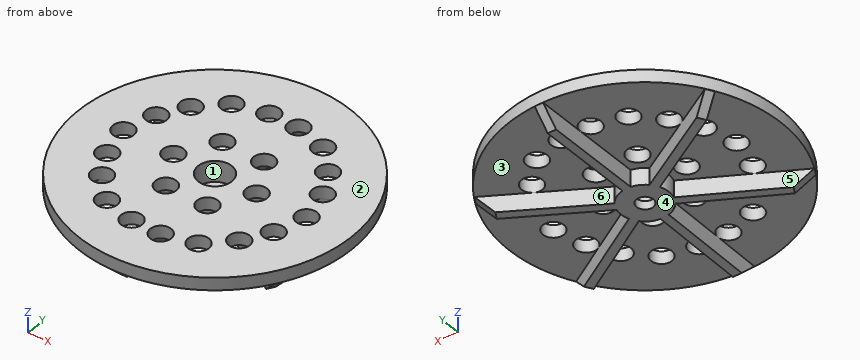
Autodesk Fusion 360 part; units mm, degrees
sketch "Skizze1" plane through (0, 0, 0) normal (0, 0, 1) x (1, 0, 0)
  circle A0 centre (0, 0) radius 32.5
  dimension "d1" = 65
extrude "Extrusion1" add sketch "Skizze1" along normal blind 3
sketch "Skizze2" plane through (0, 0, 0) normal (0, 0, -1) x (1, 0, 0)
  circle A0 centre (0, 0) radius 32.5
  circle A1 centre (0, 0) radius 5.75
  dimension "d4" = 11.5
extrude "Extrusion2" add sketch "Skizze2" along normal blind 4 contours A1
hole "Bohrung1" at (0, 0, 3) direction (0, 0, -1) diameter 4 depth 99 tip angle 118 counterbore diameter 8 counterbore depth 5
sketch "Skizze3" plane through (0, 0, 3) normal (0, 0, 1) x (-1, 0, 0)
  circle A0 centre (0, 0) radius 4
  circle A1 centre (0, 0) radius 32.5
  circle A2 centre (-10, 0.0001) radius 2.5
  circle A3 centre (-22, 0) radius 2.5
  circle A4 centre (-20, 7.5) radius 2.5
  circle A5 centre (-20, -7.5) radius 2.5
  circle A6 centre (-5, -8.6602) radius 2.5
  circle A7 centre (-16.4952, -13.5705) radius 2.5
  circle A8 centre (-11, -19.0526) radius 2.5
  circle A9 centre (-3.5048, -21.0705) radius 2.5
  circle A10 centre (5, -8.6603) radius 2.5
  circle A11 centre (3.5048, -21.0705) radius 2.5
  circle A12 centre (11, -19.0526) radius 2.5
  circle A13 centre (16.4952, -13.5705) radius 2.5
  circle A14 centre (10, -0.0001) radius 2.5
  circle A15 centre (20, -7.5) radius 2.5
  circle A16 centre (22, 0) radius 2.5
  circle A17 centre (20, 7.5) radius 2.5
  circle A18 centre (5, 8.6602) radius 2.5
  circle A19 centre (16.4952, 13.5705) radius 2.5
  circle A20 centre (11, 19.0526) radius 2.5
  circle A21 centre (3.5048, 21.0705) radius 2.5
  circle A22 centre (-5, 8.6603) radius 2.5
  circle A23 centre (-3.5048, 21.0705) radius 2.5
  circle A24 centre (-11, 19.0526) radius 2.5
  circle A25 centre (-16.4952, 13.5705) radius 2.5
  dimension "d12" = 5
  dimension "d13" = 10
  dimension "d14" = 5
  dimension "d15" = 12
  dimension "d18" = 5
  dimension "d19" = 5
  dimension "d21" = 360
extrude "Extrusion3" cut sketch "Skizze3" against normal blind 26 contours A2 | A3 | A4 | A5 | A6 | A7 | A8 | A9 | A10 | A11 | A12 | A13 | A14 | A15 | A16 | A17 | A18 | A19 | A20 | A21 | A22 | A23 | A24 | A25
sketch "Skizze4" plane through (0, 0, 0) normal (0, 0, -1) x (1, 0, 0)
  circle A0 centre (3.5048, -21.0705) radius 2.5
  circle A1 centre (22, 0) radius 2.5
  circle A2 centre (11, 19.0526) radius 2.5
  circle A3 centre (-5, -8.6603) radius 2.5
  circle A4 centre (-22, 0) radius 2.5
  circle A5 centre (-11, 19.0526) radius 2.5
  circle A6 centre (-5, 8.6602) radius 2.5
  circle A7 centre (-10, -0.0001) radius 2.5
  circle A8 centre (5, -8.6602) radius 2.5
  circle A9 centre (16.4952, 13.5705) radius 2.5
  circle A10 centre (20, -7.5) radius 2.5
  circle A11 centre (-3.5048, -21.0705) radius 2.5
  circle A12 centre (11, -19.0526) radius 2.5
  circle A13 centre (20, 7.5) radius 2.5
  circle A14 centre (10, 0.0001) radius 2.5
  circle A15 centre (-11, -19.0526) radius 2.5
  circle A16 centre (-20, 7.5) radius 2.5
  circle A17 centre (-3.5048, 21.0705) radius 2.5
  circle A18 centre (-16.4952, 13.5705) radius 2.5
  circle A19 centre (-16.4952, -13.5705) radius 2.5
  circle A20 centre (-20, -7.5) radius 2.5
  circle A21 centre (3.5048, 21.0705) radius 2.5
  circle A22 centre (16.4952, -13.5705) radius 2.5
  circle A23 centre (5, 8.6603) radius 2.5
  circle A24 centre (0, 0) radius 5.75
  circle A25 centre (0, 0) radius 32.5
  line L0 (1, -32.4807) -> (-1, -32.4807)
  line L1 (-1, -32.4807) -> (-1, -5)
  line L2 (-1, -5) -> (1, -5)
  line L3 (1, -5) -> (1, -32.4807)
  line L4 (28.6291, 15.3743) -> (4.8301, 1.634)
  line L5 (3.8301, 3.366) -> (27.6291, 17.1064)
  line L6 (27.6291, 17.1064) -> (28.6291, 15.3743)
  line L7 (4.8301, 1.634) -> (3.8301, 3.366)
  line L8 (-27.6291, 17.1064) -> (-3.8301, 3.366)
  line L9 (-4.8301, 1.634) -> (-28.6291, 15.3743)
  line L10 (-28.6291, 15.3743) -> (-27.6291, 17.1064)
  line L11 (-3.8301, 3.366) -> (-4.8301, 1.634)
  dimension "d25" = 360
extrude "Extrusion4" add sketch "Skizze4" along normal blind 4 contours A24 L4 L5 L6 | A24 L0 L1 L3 | A24 L8 L9 L10
chamfer "Fase1" distance 4 angle 45 3 edges at (0, 32.4807, -4) (28.1291, -16.2404, -4) (-28.1291, -16.2404, -4)
sketch "Skizze5" plane through (0, 0, 0) normal (0, 0, -1) x (1, 0, 0)
  circle A0 centre (3.5048, -21.0705) radius 2.5
  circle A1 centre (22, 0) radius 2.5
  circle A2 centre (11, 19.0526) radius 2.5
  circle A3 centre (-5, -8.6603) radius 2.5
  circle A4 centre (-22, 0) radius 2.5
  circle A5 centre (-11, 19.0526) radius 2.5
  circle A6 centre (-5, 8.6602) radius 2.5
  circle A7 centre (-10, -0.0001) radius 2.5
  circle A8 centre (5, -8.6602) radius 2.5
  circle A9 centre (16.4952, 13.5705) radius 2.5
  circle A10 centre (20, -7.5) radius 2.5
  circle A11 centre (-3.5048, -21.0705) radius 2.5
  circle A12 centre (11, -19.0526) radius 2.5
  circle A13 centre (20, 7.5) radius 2.5
  circle A14 centre (10, 0.0001) radius 2.5
  circle A15 centre (-11, -19.0526) radius 2.5
  circle A16 centre (-20, 7.5) radius 2.5
  circle A17 centre (-3.5048, 21.0705) radius 2.5
  circle A18 centre (-16.4952, 13.5705) radius 2.5
  circle A19 centre (-16.4952, -13.5705) radius 2.5
  circle A20 centre (-20, -7.5) radius 2.5
  circle A21 centre (3.5048, 21.0705) radius 2.5
  circle A22 centre (16.4952, -13.5705) radius 2.5
  circle A23 centre (5, 8.6603) radius 2.5
  circle A24 centre (0, 0) radius 32.5
  line L0 (-5.4038, 1.9652) -> (-28.6291, 15.3743)
  line L1 (-28.6291, 15.3743) -> (-27.6291, 17.1064)
  line L2 (-27.6291, 17.1064) -> (-4.4038, 3.6972)
  arc A25 (4.4038, 3.6972) -> (-4.4038, 3.6972) centre (0, 0) ccw
  line L3 (4.4038, 3.6972) -> (27.6291, 17.1064)
  line L4 (27.6291, 17.1064) -> (28.6291, 15.3743)
  line L5 (28.6291, 15.3743) -> (5.4038, 1.9652)
  arc A26 (1, -5.6624) -> (5.4038, 1.9652) centre (0, 0) ccw
  line L6 (1, -5.6624) -> (1, -32.4807)
  line L7 (1, -32.4807) -> (-1, -32.4807)
  line L8 (-1, -32.4807) -> (-1, -5.6624)
  arc A27 (-5.4038, 1.9652) -> (-1, -5.6624) centre (0, 0) ccw
sketch "Skizze6" plane through (0, 0, 0) normal (0, 0, -1) x (1, 0, 0)
  line L0 (5.5436, -1.6735) -> (28.5, -15.5)
  line L1 (28.5, -15.5) -> (27.4341, -17.2698)
  line L2 (27.4341, -17.2698) -> (4.4777, -3.4433)
  line L3 (4.4777, -3.4433) -> (5.5436, -1.6735)
  line L4 (-1.3225, 5.6377) -> (-0.8266, 32.4317)
  line L5 (1.239, 32.3935) -> (0.7432, 5.5995)
  line L6 (0.7432, 5.5995) -> (-1.3225, 5.6377)
  line L7 (-0.8266, 32.4317) -> (1.239, 32.3935)
  line L8 (-4.2212, -3.9642) -> (-27.6734, -16.9317)
  line L9 (-28.6731, -15.1237) -> (-5.2209, -2.1561)
  line L10 (-5.2209, -2.1561) -> (-4.2212, -3.9642)
  line L11 (-27.6734, -16.9317) -> (-28.6731, -15.1237)
  dimension "d30" = 360
extrude "Extrusion5" add sketch "Skizze6" along normal blind 4
chamfer "Fase2" distance 4 angle 45 3 edges at (-28.1733, 16.0277, -4) (27.967, 16.3849, -4) (0.2062, -32.4126, -4)
Geometry check sheet. Reference: the model listing, model coordinates, mm. Face numbers are marked on the shaded views. A direction names the side the tool comes from. Round coordinates to 2 decimals unless told otherwise and drop trailing zeros. Loops run counter-clockwise (first coordinate to the right, second up) from the corner with the lowest first, then second, coordinate; pieces in that order, holes last. Notation, with made-up numbers: M 63.5,6 L 90.5,6 A6 cw 90.5,17 Z; hole C -16,62.25 d8. An arc over 180 degrees is marked long. Return JSON: item names as keys, results as strings. Group by question number.
(1) Section check C-C, the plane x = -11. Enter the section's corners in (y, z).
(2) Section check A-A, the plane x = 16. Enter the section's corners in (y, z), and give its area (3 significant figures).
(3) Section check D-D, the plane x = 26. Enter the section's corners in (y, z), and give its area (3 significant figures).
(4) Set-up check for the marked faces 1, 2 and 3: record each of +Z, -Z, +X, -X, +Y, -Y from which the full face is reachable in a straight line by a thin tool's end or side.
(5) Scan lines: line 1 along X through (y, z) = (20.5, 0.75); line 2 along Y through (x, z) = (22, 1.35); line 3 along Y through (x, z) = (-6.5, 2.25). Record each from-to range of solid material in increasing order. Write a range as [from, to].
(6) Section check B-B, the plane z = 1.5. Give the number of separate pieces and of enclosed holes in the cut face, and give its area (3 significant figures).
(7) Mould release check, pull along Y, two halves, no side actions. Record for the marked faces 4, 5 and 6: pulls with the +Y half, pulls with the -Y half, needs draft (parallel to the pull), parting line crosses it, or undercut.
(8) Go/stop test with flat-tipped pins: pin 1 (1.5 mm diameter, centred on y = 25, z = 1, fed in from -X); pin 2 (1.2 mm diameter, centred on y = 14.5, z = -2, fed in from -X); pin 3 (4 mm diameter, centred on y = -15.5, z = 1.5, fed in from +X). Record where each tip stops, or that it passes through.
Data:
{
 "1": {"outline": "M -30.58,0 L -21.55,0 L -21.55,3 L -30.58,3 Z; M -16.55,0 L -7.51,0 L -7.51,-4 L -5.2,-4 L -5.2,0 L -2.29,0 L -2.29,3 L -16.55,3 Z; M 2.29,0 L 5.35,0 L 5.35,-4 L 7.71,-4 L 7.71,0 L 16.55,0 L 16.55,3 L 2.29,3 Z; M 21.55,0 L 30.58,0 L 30.58,3 L 21.55,3 Z"},
 "2": {"outline": "M -28.29,0 L -16.02,0 L -16.02,3 L -28.29,3 Z; M -11.12,0 L -10.39,0 L -10.39,-4 L -8.08,-4 L -8.08,0 L 7.97,0 L 7.97,-4 L 10.38,-4 L 10.38,0 L 11.12,0 L 11.12,3 L -11.12,3 Z; M 16.02,0 L 28.29,0 L 28.29,3 L 16.02,3 Z", "area": "159 mm²"},
 "3": {"outline": "M -19.5,0 L -16.17,0 L -16.17,-1.88 L -13.86,-3.04 L -13.86,0 L 13.99,0 L 13.99,-2.92 L 16.41,-1.67 L 16.41,0 L 19.5,0 L 19.5,3 L -19.5,3 Z", "area": "128 mm²"},
 "4": {"face 1": "+Z", "face 2": "+Z, +X, -X, +Y, -Y", "face 3": "-Z"},
 "5": {"line 1": "[-25.22, -13.04], [-8.96, -5.94], [-1.07, 1.07], [5.94, 8.96], [13.04, 25.22]", "line 2": "[-23.92, -9], [-6, -2.5], [2.5, 6], [9, 23.92]", "line 3": "[-31.84, -10.66], [-6.66, 6.66], [10.66, 31.84]"},
 "6": {"separate pieces": "1", "enclosed holes": "25", "area": "2,800 mm²"},
 "7": {"face 4": "needs draft", "face 5": "undercut", "face 6": "pulls with the +Y half"},
 "8": {"pin 1": "x = -21.64", "pin 2": "x = -27.45", "pin 3": "x = 29.56"}
}
